```python
from build123d import *

# Parameters (mm, degrees)
BOSS_EXTRUDE1_DEPTH = 18
CUT_EXTRUDE1_REACH  = 4
SKETCH2_R           = 6
CUT_EXTRUDE2_REACH  = 4
SKETCH3_R           = 2


with BuildPart() as part:
    # Sketch1 → Boss-Extrude1 (new body)
    with BuildSketch(Plane.XY):
        Polygon((0, 0), (0, 23), (-2, 23), (-2, 2), (-67, 2), (-67, 0), align=None)
    extrude(amount=BOSS_EXTRUDE1_DEPTH)

    # Sketch2 → Cut-Extrude1 (cut, up to next)
    with BuildSketch(Plane.ZY.offset(2), mode=Mode.PRIVATE) as cut_extrude1_sk1:
        with Locations((9, 15)):
            Circle(SKETCH2_R)
    cut_extrude1_tool1 = extrude(cut_extrude1_sk1.sketch, amount=-CUT_EXTRUDE1_REACH, mode=Mode.PRIVATE) & part.part
    add(cut_extrude1_tool1.solids().sort_by_distance((-2, 15, 9))[0], mode=Mode.SUBTRACT)

    # Sketch3 → Cut-Extrude2 (cut, up to next)
    with BuildSketch(Plane(origin=(0, 2, 0), x_dir=(1, 0, 0), z_dir=(0, 1, 0)), mode=Mode.PRIVATE) as cut_extrude2_sk1:
        with Locations((-63, -9)):
            Circle(SKETCH3_R)
    cut_extrude2_tool1 = extrude(cut_extrude2_sk1.sketch, amount=-CUT_EXTRUDE2_REACH, mode=Mode.PRIVATE) & part.part
    add(cut_extrude2_tool1.solids().sort_by_distance((-63, 2, 9))[0], mode=Mode.SUBTRACT)
    # Sketch3 → Cut-Extrude2 (cut, up to next)
    with BuildSketch(Plane(origin=(0, 2, 0), x_dir=(1, 0, 0), z_dir=(0, 1, 0)), mode=Mode.PRIVATE) as cut_extrude2_sk2:
        with Locations((-53, -9)):
            Circle(SKETCH3_R)
    cut_extrude2_tool2 = extrude(cut_extrude2_sk2.sketch, amount=-CUT_EXTRUDE2_REACH, mode=Mode.PRIVATE) & part.part
    add(cut_extrude2_tool2.solids().sort_by_distance((-53, 2, 9))[0], mode=Mode.SUBTRACT)


solid = part.part
```
The listing builds one solid part. Answer for the finished solid, in the listing's coordinates (mm). A direction names the side the tool comes from. Give positions to 0.01 mm unless a question says otherwise; leave off trailing zeros. Loops run counter-clockwise (first coordinate to the right, second up) from the corner with the lowest first, then second, coordinate; pieces in that order, holes last. Notation, with made-up numbers: M -17.75,-7 L 18.25,-7 A19 ccw 18.25,7 Z; hole C 27,-5 d4. An arc over 180 degrees is marked long. One line per item, written item: value.
Q1. A cutting plane is placed at D-D on y = 7.5. Determine the outline of the cut face in (x, z), then the cut area to 3 significant figures.
Working result:
outline: M -2,0 L 0,0 L 0,18 L -2,18 Z
area: 36.0 mm^2
Q2. A cutting plane is placed at B-B on x = -53. Determine the outline of the cut face in (y, z).
Working result:
outline: M 0,0 L 2,0 L 2,7 L 0,7 Z; M 0,11 L 2,11 L 2,18 L 0,18 Z
Q3. Flat-ended cylindrical pins translate along their axes: P1, Ø10, axis at y = 3.5, z = 13, coming from the +X side; P2, Ø10, axis at x = -43.5, z = 16, coming from the +Y side; P3, Ø3.5, axis at x = -53, z = 9, coming from the -Y side; P4, Ø6, axis at y = 8, z = 7.5, coming from the -X side. Find the tip coordinate at first contact, or state that the pin passes through.
Working result:
P1: stops at x = 0
P2: stops at y = 2
P3: passes through
P4: stops at x = -2
Q4. Determine the mould class of faces 3 (the face through (0, 8.8, 8.9)), 4 (the face through (-67, 1, 9)), 5 (the face through (-54.474, 1.014, 7.648)) for opening direction X: +X half, -X half, draft (parallel to the pull), parting line (faces both ways), or undercut.
Working result:
face 3: +X half
face 4: -X half
face 5: undercut
Q5. A cutting plane is placed at A-A on y = 15. Determine the outline of the cut face in (x, z), then the cut area to 3 significant figures.
Working result:
outline: M -2,0 L 0,0 L 0,3 L -2,3 Z; M -2,15 L 0,15 L 0,18 L -2,18 Z
area: 12.0 mm^2
Q6. Find the intervals of material crossed by line 1 (X direction, y = 1.45, z = 9); line 2 (Y direction, x = -1.35, z = 9); line 3 (Z direction, x = -63, y = 1.1), in increasing order. Write a range as from..to.
Working result:
line 1: x = -67..-65, -61..-55, -51..0
line 2: y = 0..9, 21..23
line 3: z = 0..7, 11..18
Q7. For faces 1 (the face through (-64.474, 1.014, 7.648)), 2 (the face through (-34, 2, 9)), determine the directions among +Z, -Z, +X, -X, +Y, -Y from which every point of the face is accessible in a straight line to the end or side of a thin tool.
Working result:
face 1: +Y, -Y
face 2: +Z, -Z, -X, +Y
Q8. A cutting plane is placed at C-C on z = 6. Determine the outline of the cut face in (x, y), then the cut area to 3 significant figures.
Working result:
outline: M -67,0 L 0,0 L 0,9.8 L -2,9.8 L -2,2 L -67,2 Z; M -2,20.2 L 0,20.2 L 0,23 L -2,23 Z
area: 155 mm^2
